Geometry check sheet. Reference: drawing and pictorial views, mm from the part's lowest x, y, z. A direction names the side the tool comes from. Give positions to 0.01 mm unless a question says otherwise; leave off trailing zeros. Write each loop counter-clockwise with the first axis right and the second up, starting at its lowest first coordinate (ties: lowest second). Pieces come first, ordered by that corner, then holes. Notation, with made-up numbers: M 27.5,-15 L 85.5,-15 A17 cw 85.5,10 Z; hole C 8,-13.5 d5. An arc over 180 degrees is marked long. One line per item, written item: value. Start each with the question number.
1. Scan lines: line 1 (X direction, y = 2.25, z = 4.25); line 2 (Z direction, x = 8.75, y = 9.5); line 3 (Y direction, x = 15.75, z = 6.25). Record each from-to range of solid material in increasing order.
2. Cross-section at D-D on x = 1.5. Record the cut outline in (y, z) (1 decimal).
3. Gauge pin test, flat ends, axial feed: pin 1 (4 mm diameter, centred on x = 11, z = 6, fed in from +Y); pin 2 (2.5 mm diameter, centred on x = 10.5, z = 4, fed in from -Y); pin 3 (3 mm diameter, centred on x = 4.5, y = 7, fed in from +Z); pin 4 (1.5 mm diameter, centred on x = 3.5, z = 7, fed in from +Y). Record the tip position at first contact, or that the pin passes through.
4. Cross-section at C-C on y = 8. Record the cut outline in (x, z) (1 decimal).
5. Cross-section at B-B on x = 12. Record the cut outline in (y, z).
6. Tool access check on the marked faces 1, 2, 3 and 4. Record the directions out of +Z, -Z, +X, -X, +Y, -Y that give a thin tool (end or side, any length) a straight path to the whole face; none if there is none.
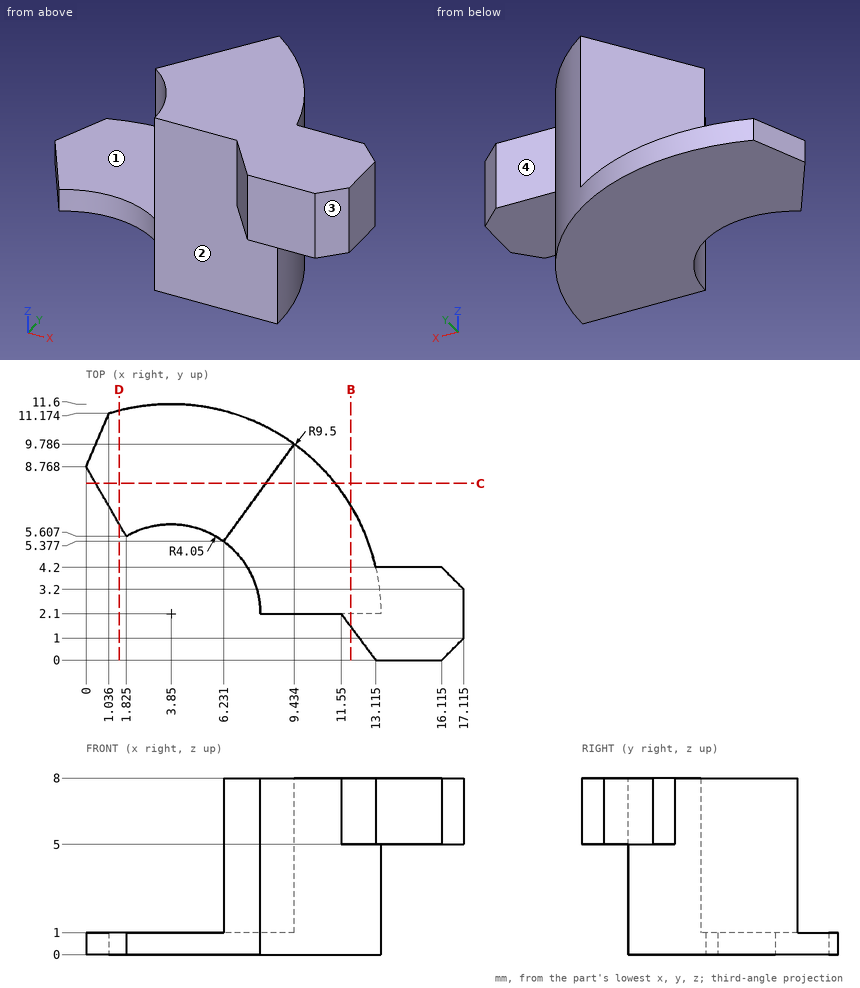
Report:
1. line 1: x = 7.9 to 13.35
1. line 2: z = 0 to 1
1. line 3: y = 0 to 4.2
2. outline: M 6.2,0 L 11.3,0 L 11.3,1 L 6.2,1 Z
3. pin 1: stops at y = 9.79
3. pin 2: stops at y = 2.1
3. pin 3: stops at z = 1
3. pin 4: passes through
4. outline: M 0.4,0 L 11.3,0 L 11.3,8 L 8.1,8 L 8.1,1 L 0.4,1 Z
5. outline: M 1.5,5 L 2.1,5 L 2.1,0 L 6.98,0 L 6.98,8 L 1.5,8 Z
6. face 1: +Z, -X, +Y
6. face 2: -Z, -X, -Y
6. face 3: +Z, -Z, +X, -Y
6. face 4: +Z, -Z, +X, +Y
